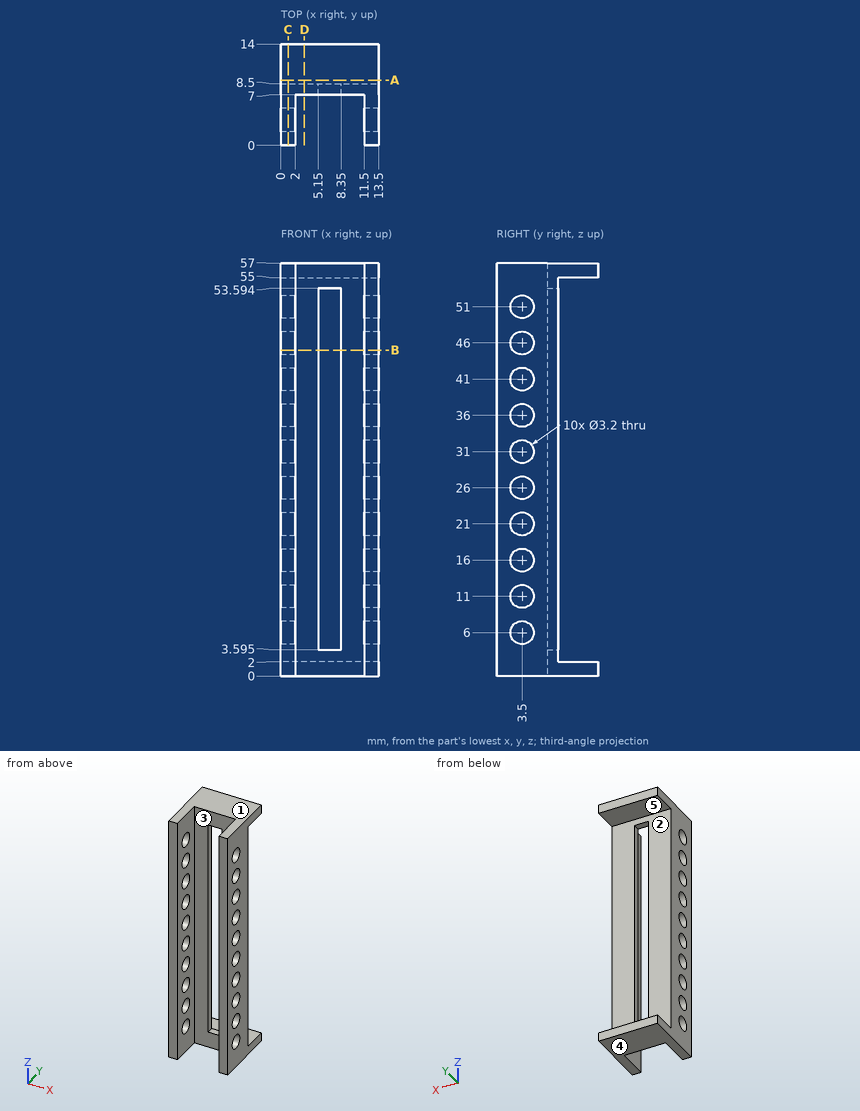
Could you check a few things on this drawing? It's one solid part, dimensions in mm from its lowest x, y, z. A direction names the side the tool comes from. Give positions to 0.01 mm unless a question says otherwise; leave off trailing zeros. Order: outer loops, then holes, each group sorted by start corner. A loop starts at its lowest first (then second) coordinate and runs counter-clockwise, first axis right, second up.
1. Suppose I cut it at D-D (x = 3.25). Write out the boundary of the cut face in (y, z).
Answers below:
outline: (7, 0) - (14, 0) - (14, 2) - (8.5, 2) - (8.5, 55) - (14, 55) - (14, 57) - (7, 57) - close
2. I need wall thicknesses on L1, parallel to Z at x = 10.25, y = 10.75; L2, parallel to Y at x = 1.3, z = 26; L3, parallel to X at y = 3, z = 44. Which ranges of each line are inside material? Lowest first, please.
Answers below:
L1: z = 0 to 2, 55 to 57
L2: y = 0 to 1.9, 5.1 to 8.5
L3: x = 0 to 2, 11.5 to 13.5
3. Which directions (+Z, -Z, +X, -X, +Y, -Y) give clear straight access to the entire face, cutting with the end or side of a thin tool? Please do the marked faces 1 and 2.
Answers below:
face 1: +Z, +X, -X, +Y, -Y
face 2: +X, -X, +Y
4. Suppose I cut it at B-B (z = 45). Write out the boundary of the cut face in (x, y).
Answers below:
outline: (0, 0) - (2, 0) - (2, 2.25) - (0, 2.25) - close; (0, 4.75) - (2, 4.75) - (2, 7) - (5.15, 7) - (5.15, 8.5) - (0, 8.5) - close; (8.35, 7) - (11.5, 7) - (11.5, 4.75) - (13.5, 4.75) - (13.5, 8.5) - (8.35, 8.5) - close; (11.5, 0) - (13.5, 0) - (13.5, 2.25) - (11.5, 2.25) - close
5. For pin 1 (5 mm diameter, centred on y = 3.5, z = 6, fed in from +X); pin 2 (3 mm diameter, centred on x = 10, z = 39.5, fed in from +Y); pin 3 (1 mm diameter, centred on x = 10, z = 22, fed in from -Y), each with a flat end and sliding along its axis, tell me the tip position at first contact or that it passes through.
Answers below:
pin 1: stops at x = 13.5
pin 2: stops at y = 8.5
pin 3: stops at y = 7
6. Suppose I cut it at A-A (y = 9). Write out the boundary of the cut face in (x, z).
Answers below:
outline: (0, 0) - (13.5, 0) - (13.5, 2) - (0, 2) - close; (0, 55) - (13.5, 55) - (13.5, 57) - (0, 57) - close
7. Suppose I cut it at C-C (x = 1). State how many separate pieces and enclosed holes the cut face has, plus the area to 3 significant figures.
Answers below:
separate pieces: 1
enclosed holes: 10
area: 426 mm2
8. Thinking about a two-plate mould opening in Z: for the marked faces 3, 4 and 5, which applies, +Z half, -Z half, draft (parallel to the pull), parting line (faces both ways), or undercut?
Answers below:
face 3: draft
face 4: -Z half
face 5: undercut
